Could you check a few things on this model? Use its own coordinates, in mm. A direction names the side the tool comes from. Round coordinates to 2 decimals unless told otherwise and drop trailing zeros. Order: outer loops, then holes, each group sorted by start corner. A loop starts at its lowest first (then second) coordinate and runs counter-clockwise, first axis right, second up. Notation, with made-up numbers: (62, -8) - (82, -8) arc R27 cw to (82, 8) - close; hole circle Ø2 at (-40, 29). An arc over 180 degrees is marked (long way). Use one line per item in the form item = value.
from build123d import *

# Parameters (mm, degrees)
F0_R     = 6.25
F1_DEPTH = 12.5
F3_R     = 2.5
F3_R_2   = 7.5
F4_REACH = 159.0869091096


with BuildPart() as f1:
    # F0 (on Top) → F1 (new body)
    with BuildSketch(Plane.XY):
        with BuildLine():
            Line((0, 32), (0, 6.5))
            Line((0, 6.5), (13, 6.5))
            ThreePointArc((13, 6.5), (19.5, 0), (13, -6.5))
            Line((13, -6.5), (0, -6.5))
            Line((0, -6.5), (0, -32))
            ThreePointArc((0, -32), (13, -45), (26, -32))
            Line((26, -32), (26, -20.1084308683))
            Line((26, -20.1084308683), (90, -20.1084308683))
            Line((90, -20.1084308683), (90, -32))
            ThreePointArc((90, -32), (103, -45), (116, -32))
            Line((116, -32), (116, 32))
            ThreePointArc((116, 32), (103, 45), (90, 32))
            Line((90, 32), (90, 20.1084308683))
            Line((90, 20.1084308683), (26, 20.1084308683))
            Line((26, 20.1084308683), (26, 32))
            ThreePointArc((26, 32), (13, 45), (0, 32))
        make_face()
        with Locations((13, -32)):
            Circle(F0_R, mode=Mode.SUBTRACT)
        with Locations((103, -32)):
            Circle(F0_R, mode=Mode.SUBTRACT)
        with Locations((13, 32)):
            Circle(F0_R, mode=Mode.SUBTRACT)
        with Locations((103, 32)):
            Circle(F0_R, mode=Mode.SUBTRACT)
    extrude(amount=F1_DEPTH)

    f4_end = f1.faces().sort_by_distance((59.8447932422, 0, 0))[0]
    # F3 (on face) → F4 (join, up to a face of the model that its end follows)
    with BuildSketch(Plane(origin=(64.25, 0, 64.25), x_dir=(0, -1, 0), z_dir=(-0.7071067812, 0, -0.7071067812))):
        with BuildLine():
            Line((-20.1084308683, -73.1855518528), (20.1084308683, -73.1855518528))
            Line((20.1084308683, -73.1855518528), (20.1084308683, -38.1855518528))
            ThreePointArc((20.1084308683, -38.1855518528), (0, -18.0771209845), (-20.1084308683, -38.1855518528))
            Line((-20.1084308683, -38.1855518528), (-20.1084308683, -73.1855518528))
        make_face()
        with Locations((-7.3473156537, -48.2982642825)):
            Circle(F3_R, mode=Mode.SUBTRACT)
        with Locations((7.3473156537, -48.2982642825)):
            Circle(F3_R, mode=Mode.SUBTRACT)
        with Locations((-11.8882064537, -34.3228394231)):
            Circle(F3_R, mode=Mode.SUBTRACT)
        with Locations((0, -38.1855518528)):
            Circle(F3_R_2, mode=Mode.SUBTRACT)
        with Locations((11.8882064537, -34.3228394231)):
            Circle(F3_R, mode=Mode.SUBTRACT)
        with Locations((0, -25.6855518528)):
            Circle(F3_R, mode=Mode.SUBTRACT)
    f4_long = extrude(amount=F4_REACH, mode=Mode.PRIVATE)
    add(split(f4_long, bisect_by=f4_end, keep=Keep.BOTTOM, mode=Mode.PRIVATE))


solid = f1.part
Item 1: Imagine slicing it at C-C on y = 34. Please give me the cut outline in (x, z), plus the area to 3 significant figures.
Found:
outline = (0.15, 0) - (7.08, 0) - (7.08, 12.5) - (0.15, 12.5) - close; (18.92, 0) - (25.85, 0) - (25.85, 12.5) - (18.92, 12.5) - close; (90.15, 0) - (97.08, 0) - (97.08, 12.5) - (90.15, 12.5) - close; (108.92, 0) - (115.85, 0) - (115.85, 12.5) - (108.92, 12.5) - close
area = 346 mm2
Item 2: If we mould it in two halves opening along Y, with no side actions, what happens to faces 1 (the face through (8.39, -27.78, 6.16)), 2 (the face through (103, -45, 6)), 3 (the face through (57, 1, 0))? For each: released by +Y, released by -Y, zero draft, split by the parting line, or undercut.
Found:
face_1 = undercut
face_2 = released by -Y
face_3 = zero draft
Item 3: I need wall thicknesses on L1, parallel to X at y = -5.5, z = 16; L2, parallel to Y at x = 103, z = 4.25; L3, parallel to Y at x = 13, z = 4.5. Which ranges of each line are inside material? Lowest first, please.
Found:
L1 = 42.65 to 62.79, 77.21 to 81.92, 86.69 to 112.5
L2 = -45 to -38.25, -25.75 to 25.75, 38.25 to 45
L3 = -45 to -38.25, -25.75 to -6.5, 6.5 to 25.75, 38.25 to 45
Item 4: Imagine slicing it at B-B on x = 103. Please give me the cut outline in (y, z).
Found:
outline = (-45, 0) - (-38.25, 0) - (-38.25, 12.5) - (-45, 12.5) - close; (-25.75, 0) - (25.75, 0) - (25.75, 12.5) - (20.11, 12.5) - (20.11, 25.5) - (-20.11, 25.5) - (-20.11, 12.5) - (-25.75, 12.5) - close; (38.25, 0) - (45, 0) - (45, 12.5) - (38.25, 12.5) - close
Item 5: Will these pins go through, and if not, where does the flat tip stop? P1, Ø1.5, axis at x = 80, z = 6.5, coming from the -Y side; P2, Ø10, axis at x = 44, z = 6.5, coming from the +Y side; P3, Ø8, axis at x = 95, y = 16, coming from the +Z side; P4, Ø4, axis at y = -32.5, z = 15.5, coming from the +X side.
Found:
P1 = -20.11
P2 = 20.11
P3 = 37.5
P4 = through
Item 6: Imagine slicing it at A-A on y = 23. Please give me the cut outline in (x, z).
Found:
outline = (0, 0) - (26, 0) - (26, 12.5) - (0, 12.5) - close; (90, 0) - (116, 0) - (116, 12.5) - (90, 12.5) - close
Item 7: Imagine slicing it at D-D on z = 14. State how many separate pieces and enclosed holes the cut face has, plus the area to 3 significant figures.
Found:
separate_pieces = 1
enclosed_holes = 6
area = 2,380 mm2
Item 8: For faces 4 (the face through (90, -26, 6)), 5 (the face through (81, -7, 12.5)), 6 (the face through (6, 6.5, 6)), which set-ups out of +Z, -Z, +X, -X, +Y, -Y let a thin tool reach every point of the face, with its end or its side?
Found:
face_4 = +Z, -Z, -Y
face_5 = none
face_6 = +Z, -Z, -X
